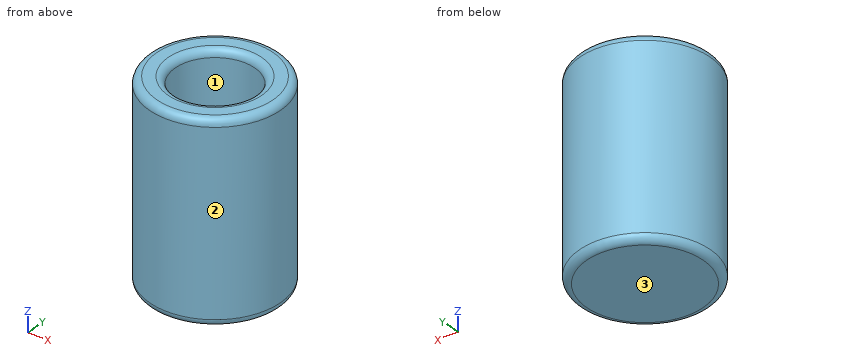
```python
from build123d import *


with BuildPart() as f1:
    # F0 (on Front) → F1 (revolve)
    with BuildSketch(Plane.XZ):
        with BuildLine():
            ThreePointArc((-16.265942, 37.24327), (-17.702014, 36.669703), (-18.299835, 35.243557))
            Line((-18.299835, 35.243557), (-18.299835, -14.91217))
            ThreePointArc((-18.299835, -14.91217), (-17.714048, -16.326383), (-16.299835, -16.91217))
            Line((-16.299835, -16.91217), (0, -16.91217))
            Line((0, -16.91217), (0, -8.116585))
            Line((0, -8.116585), (-9.116645, -8.116585))
            ThreePointArc((-9.116645, -8.116585), (-10.530858, -7.530798), (-11.116645, -6.116585))
            Line((-11.116645, -6.116585), (-11.116645, 35.189605))
            ThreePointArc((-11.116645, 35.189605), (-11.690498, 36.591784), (-13.082751, 37.189318))
            Line((-13.082751, 37.189318), (-16.265942, 37.24327))
        make_face()
    revolve(axis=Axis((0, 0, 10.792887), (0, 0, -1)))


solid = f1.part
```
The model under review builds one solid part; all positions refer to its coordinate system, in mm. Face numbers are marked on the shaded views. Give positions to 0.01 mm unless a question says otherwise; leave off trailing zeros. Write each loop counter-clockwise with the first axis right and the second up, starting at its lowest first coordinate (ties: lowest second). Pieces come first, ordered by that corner, then holes. Notation, with made-up numbers: (-3, 57) - (46, 57) arc R17 cw to (46, 75) - close; hole circle Ø11 at (-14, 52.25). An arc over 180 degrees is marked (long way). Answer in a Markdown table with one row per item. Add a question column.
1. Draft analysis for pull direction X (two halves, no side actions). For the marked faces 1, 2 and 3, state which applies: +X half, -X half, draft (parallel to the pull), parting line (faces both ways), or undercut.
2. We need section A-A on z = 33.5. Write out the cut boundary in (x, y), then the cut area to 3 significant figures.
3. Insertion check: P1, Ø4, axis at x = 1, y = 1.5, coming from the +Z side; P2, Ø2, axis at x = 8, z = 11, coming from the +Y side; P3, Ø14.5, axis at x = 3, y = 1.5, coming from the +Z side. Each pin has a flat end and moves straight along its axis. Give the tip position at first contact, or say it passes through.
4. Wall thickness on line 1 along Y through (x, z) = (0, 19); line 2 along Z through (x, y) = (-2, 0.5); line 3 along Z through (x, y) = (-12, 6): over which ranges is each line inside the solid? List them lowest first. Write a range as [from, to].
5. We need section B-B on x = 0. Write out the cut boundary in (y, z), then the cut area to 3 significant figures.
Ans:
| question | item | result |
|---|---|---|
| 1 | face 1 | undercut |
| 1 | face 2 | parting line |
| 1 | face 3 | draft |
| 2 | outline | circle Ø36.6 at (0, 0); hole circle Ø22.23 at (0, 0) |
| 2 | area | 664 mm^2 |
| 3 | P1 | stops at z = -8.12 |
| 3 | P2 | stops at y = 16.91 |
| 3 | P3 | stops at z = -7.45 |
| 4 | line 1 | y = [-18.3, -11.12], [11.12, 18.3] |
| 4 | line 2 | z = [-16.91, -8.12] |
| 4 | line 3 | z = [-16.91, 37.19] |
| 5 | outline | (-18.3, -14.91) arc R2 ccw to (-16.3, -16.91) - (16.3, -16.91) arc R2 ccw to (18.3, -14.91) - (18.3, 35.24) arc R2 ccw to (16.27, 37.24) - (13.08, 37.19) arc R2 ccw to (11.12, 35.19) - (11.12, -6.12) arc R2 cw to (9.12, -8.12) - (-9.12, -8.12) arc R2 cw to (-11.12, -6.12) - (-11.12, 35.19) arc R2 ccw to (-13.08, 37.19) - (-16.27, 37.24) arc R2 ccw to (-18.3, 35.24) - close |
| 5 | area | 970 mm^2 |
